Part model, mm, in its own coordinate system. A direction names the side the tool comes from. Give positions to 0.01 mm unless a question says otherwise; leave off trailing zeros. Order: outer loops, then holes, each group sorted by start corner. A loop starts at its lowest first (then second) coordinate and runs counter-clockwise, first axis right, second up. Notation, with made-up numbers: (52.25, 10.5) - (77.25, 10.5) arc R15 cw to (77.25, 28.5) - close; hole circle Ø3 at (49.5, 67.5). An arc over 180 degrees is marked (long way). One line per item, written item: value.
```python
from build123d import *

# Parameters (mm, degrees)
BOSS_EXTRUDE1_DEPTH                  = 194
BOSS_EXTRUDE1_DEPTH_BACK             = 194
TAP_DRILL_FOR_M5X0_8_TAP1_D          = 4.2
TAP_DRILL_FOR_M5X0_8_TAP1_DEPTH      = 3.048
TAP_DRILL_FOR_M3X0_5_TAP1_D          = 2.5
TAP_DRILL_FOR_M3X0_5_TAP1_DEPTH      = 3.048
TAP_DRILL_FOR_M5X0_8_TAP2_AT_2_COUNT = 2
TAP_DRILL_FOR_M5X0_8_TAP2_AT_2_PITCH = 25.4
BOSS_EXTRUDE3_START                  = 40
BOSS_EXTRUDE3_DEPTH                  = 40
M5_CLEARANCE_HOLE1_D                 = 5.3
M5_CLEARANCE_HOLE1_DEPTH             = 3.048
BOSS_EXTRUDE4_START                  = 7
BOSS_EXTRUDE4_DEPTH                  = 7
F_8_0_8_DIAMETER_HOLE1_D             = 8
F_8_0_8_DIAMETER_HOLE1_DEPTH         = 3.048
F_8_0_8_DIAMETER_HOLE2_D             = 8
F_8_0_8_DIAMETER_HOLE2_DEPTH         = 3.048


with BuildPart() as part:
    # Sketch4 → Boss-Extrude1 (new, two sides: drawn at the far end of the back side and taken through both)
    with BuildSketch(Plane(origin=(0, 0, 0), x_dir=(0, 0, -1), z_dir=(1, 0, 0)).offset(-BOSS_EXTRUDE1_DEPTH_BACK)):
        with BuildLine():
            Line((19.05, -17.145), (19.05, 17.145))
            ThreePointArc((19.05, 17.145), (18.492038418, 18.492038418), (17.145, 19.05))
            Line((17.145, 19.05), (-17.145, 19.05))
            ThreePointArc((-17.145, 19.05), (-18.492038418, 18.492038418), (-19.05, 17.145))
            Line((-19.05, 17.145), (-19.05, -17.145))
            ThreePointArc((-19.05, -17.145), (-18.492038418, -18.492038418), (-17.145, -19.05))
            Line((-17.145, -19.05), (17.145, -19.05))
            ThreePointArc((17.145, -19.05), (18.492038418, -18.492038418), (19.05, -17.145))
        make_face()
        with BuildLine():
            Line((16.002, 14.4018), (16.002, -14.4018))
            ThreePointArc((16.002, -14.4018), (15.533312271, -15.533312271), (14.4018, -16.002))
            Line((14.4018, -16.002), (-14.4018, -16.002))
            ThreePointArc((-14.4018, -16.002), (-15.533312271, -15.533312271), (-16.002, -14.4018))
            Line((-16.002, -14.4018), (-16.002, 14.4018))
            ThreePointArc((-16.002, 14.4018), (-15.533312271, 15.533312271), (-14.4018, 16.002))
            Line((-14.4018, 16.002), (14.4018, 16.002))
            ThreePointArc((14.4018, 16.002), (15.533312271, 15.533312271), (16.002, 14.4018))
        make_face(mode=Mode.SUBTRACT)
    extrude(amount=BOSS_EXTRUDE1_DEPTH + BOSS_EXTRUDE1_DEPTH_BACK)

    # Tap Drill for M5x0.8 Tap1
    with Locations(Plane(origin=(0, 19.05, 0), x_dir=(1, 0, 0), z_dir=(0, 1, 0))):
        with Locations((-126, 7.05), (-126, -10.95)):
            tap_drill_for_m5x0_8_tap1 = Hole(TAP_DRILL_FOR_M5X0_8_TAP1_D / 2, depth=TAP_DRILL_FOR_M5X0_8_TAP1_DEPTH)

    # Tap Drill for M3x0.5 Tap1
    with Locations(Plane.XY.offset(19.05)):
        with Locations((149, 9.05), (89, 9.05), (29, 9.05), (-31, 9.05), (-91, 9.05), (-61, 9.05)):
            tap_drill_for_m3x0_5_tap1 = Hole(TAP_DRILL_FOR_M3X0_5_TAP1_D / 2, depth=TAP_DRILL_FOR_M3X0_5_TAP1_DEPTH)

    # Sketch22 → Tap Drill for M5x0.8 Tap2 (revolve, cut)
    with BuildSketch(Plane(origin=(174.95, 12.7, 19.05), x_dir=(0, -1, 0), z_dir=(1, 0, 0))):
        Polygon((0, 0), (0, 6.2618073), (2.1, 5), (2.1, 0), align=None)
    tap_drill_for_m5x0_8_tap2 = revolve(axis=Axis((174.95, 12.7, 25.4), (0, 0, -1)), mode=Mode.SUBTRACT)

    # Tap Drill for M5x0.8 Tap2 at 2: Tap Drill for M5x0.8 Tap2 ×2
    with Locations(*[(0, -i * TAP_DRILL_FOR_M5X0_8_TAP2_AT_2_PITCH, 0) for i in range(1, TAP_DRILL_FOR_M5X0_8_TAP2_AT_2_COUNT)]):
        add(tap_drill_for_m5x0_8_tap2, mode=Mode.SUBTRACT)

    # Mirror1: Tap Drill for M5x0.8 Tap1, Tap Drill for M3x0.5 Tap1, Tap Drill for M5x0.8 Tap2 across plane
    add(tap_drill_for_m5x0_8_tap1.mirror(Plane(origin=(0, 0, 0), x_dir=(0, 0.7071067811865478, 0.7071067811865472), z_dir=(0, -0.7071067811865475, 0.7071067811865477))), mode=Mode.SUBTRACT)
    add(tap_drill_for_m3x0_5_tap1.mirror(Plane(origin=(0, 0, 0), x_dir=(0, 0.7071067811865478, 0.7071067811865472), z_dir=(0, -0.7071067811865475, 0.7071067811865477))), mode=Mode.SUBTRACT)
    add(tap_drill_for_m5x0_8_tap2.mirror(Plane(origin=(0, 0, 0), x_dir=(0, 0.7071067811865478, 0.7071067811865472), z_dir=(0, -0.7071067811865475, 0.7071067811865477))), mode=Mode.SUBTRACT)

    # Mirror1 copy 1 sketch → Mirror1 copy 1 (revolve, cut)
    with BuildSketch(Plane(origin=(174.95, 19.05, -12.7), x_dir=(0, 0, -1), z_dir=(1, 0, 0))):
        Polygon((0, 0), (0, -6.2618073), (2.1, -5), (2.1, 0), align=None)
    revolve(axis=Axis((174.95, 25.4, -12.7), (0, 1, 0)), mode=Mode.SUBTRACT)

    # Sketch11 → Boss-Extrude3 (add)
    with BuildSketch(Plane.ZY.offset(194).offset(BOSS_EXTRUDE3_START)):
        with BuildLine():
            Line((-17.145, -19.05), (17.145, -19.05))
            ThreePointArc((17.145, -19.05), (18.492038418, -18.492038418), (19.05, -17.145))
            Line((19.05, -17.145), (19.05, 17.145))
            ThreePointArc((19.05, 17.145), (18.492038418, 18.492038418), (17.145, 19.05))
            Line((17.145, 19.05), (-17.145, 19.05))
            ThreePointArc((-17.145, 19.05), (-18.492038418, 18.492038418), (-19.05, 17.145))
            Line((-19.05, 17.145), (-19.05, -17.145))
            ThreePointArc((-19.05, -17.145), (-18.492038418, -18.492038418), (-17.145, -19.05))
        make_face()
        with BuildLine():
            Line((-16.002, 14.4018), (-16.002, -14.4018))
            ThreePointArc((-16.002, -14.4018), (-15.533312271, -15.533312271), (-14.4018, -16.002))
            Line((-14.4018, -16.002), (14.4018, -16.002))
            ThreePointArc((14.4018, -16.002), (15.533312271, -15.533312271), (16.002, -14.4018))
            Line((16.002, -14.4018), (16.002, 14.4018))
            ThreePointArc((16.002, 14.4018), (15.533312271, 15.533312271), (14.4018, 16.002))
            Line((14.4018, 16.002), (-14.4018, 16.002))
            ThreePointArc((-14.4018, 16.002), (-15.533312271, 15.533312271), (-16.002, 14.4018))
        make_face(mode=Mode.SUBTRACT)
    extrude(amount=-BOSS_EXTRUDE3_DEPTH)

    # M5 Clearance Hole1
    with Locations(Plane(origin=(0, 19.05, 0), x_dir=(1, 0, 0), z_dir=(0, 1, 0))):
        with Locations((-229, 6.8), (-229, -6.95), (-184, -6.95), (-184, 6.8)):
            m5_clearance_hole1 = Hole(M5_CLEARANCE_HOLE1_D / 2, depth=M5_CLEARANCE_HOLE1_DEPTH)

    # Mirror2: M5 Clearance Hole1 across plane
    add(m5_clearance_hole1.mirror(Plane(origin=(0, 0, 0), x_dir=(0, 0.7071067811865478, 0.7071067811865472), z_dir=(0, -0.7071067811865475, 0.7071067811865477))), mode=Mode.SUBTRACT)

    # Sketch16 → Boss-Extrude4 (add)
    with BuildSketch(Plane.ZY.offset(234).offset(BOSS_EXTRUDE4_START)):
        with BuildLine():
            Line((-17.145, -19.05), (17.145, -19.05))
            ThreePointArc((17.145, -19.05), (18.492038418, -18.492038418), (19.05, -17.145))
            Line((19.05, -17.145), (19.05, 17.145))
            ThreePointArc((19.05, 17.145), (18.492038418, 18.492038418), (17.145, 19.05))
            Line((17.145, 19.05), (-17.145, 19.05))
            ThreePointArc((-17.145, 19.05), (-18.492038418, 18.492038418), (-19.05, 17.145))
            Line((-19.05, 17.145), (-19.05, -17.145))
            ThreePointArc((-19.05, -17.145), (-18.492038418, -18.492038418), (-17.145, -19.05))
        make_face()
        with BuildLine():
            Line((-16.002, 14.4018), (-16.002, -14.4018))
            ThreePointArc((-16.002, -14.4018), (-15.533312271, -15.533312271), (-14.4018, -16.002))
            Line((-14.4018, -16.002), (14.4018, -16.002))
            ThreePointArc((14.4018, -16.002), (15.533312271, -15.533312271), (16.002, -14.4018))
            Line((16.002, -14.4018), (16.002, 14.4018))
            ThreePointArc((16.002, 14.4018), (15.533312271, 15.533312271), (14.4018, 16.002))
            Line((14.4018, 16.002), (-14.4018, 16.002))
            ThreePointArc((-14.4018, 16.002), (-15.533312271, 15.533312271), (-16.002, 14.4018))
        make_face(mode=Mode.SUBTRACT)
    extrude(amount=-BOSS_EXTRUDE4_DEPTH)

    # Ø8.0 (8) Diameter Hole1
    with Locations(Plane.XY.offset(-16.002)):
        with Locations((-229, -6.8), (-229, 6.95), (-184, 6.95), (-184, -6.8)):
            Hole(F_8_0_8_DIAMETER_HOLE1_D / 2, depth=F_8_0_8_DIAMETER_HOLE1_DEPTH)

    # Ø8.0 (8) Diameter Hole2
    with Locations(Plane(origin=(0, -16.002, 0), x_dir=(1, 0, 0), z_dir=(0, 1, 0))):
        with Locations((-229, 6.8), (-229, -6.95), (-184, -6.95), (-184, 6.8)):
            Hole(F_8_0_8_DIAMETER_HOLE2_D / 2, depth=F_8_0_8_DIAMETER_HOLE2_DEPTH)


solid = part.part
```
1) Pin check, flat tips, straight feed: pin 1 (2 mm diameter, centred on x = 149, y = 9.05, fed in from +Z); pin 2 (7 mm diameter, centred on x = -229, y = 6.95, fed in from -Z); pin 3 (7 mm diameter, centred on x = -184, z = 6.95, fed in from -Y). Stop position of each tip, or through.
Outcome:
pin 1: stops at z = -16
pin 2: stops at z = 16
pin 3: stops at y = 16
2) Mould opens along X. For faces 6 (the flat face through (-27, 0, 16.002)), 7 (the flat face through (194, 0, 17)), 8 (the cylindrical face through (-187.815, -17.547, -8.001)) say: released by +X, released by -X, zero draft, split by the parting line, or undercut.
Outcome:
face 6: zero draft
face 7: released by +X
face 8: undercut
3) Drill centre lines: line 1 along Y through (x, z) = (-229, 17); line 2 along Z through (x, y) = (-106.5, 8). Where is each one in solid material? Low to high. Write a range as from..to.
Outcome:
line 1: y = -19.05..-9.45, -4.15..4.3, 9.6..19.05
line 2: z = -19.05..-16, 16..19.05
4) Which spindle directions (+Z, -Z, +X, -X, +Y, -Y) get a long thin tool onto all of the face, cutting with end or side? Do faces 1 (the cylindrical face through (-225, -18, 7)), 2 (the flat face through (-27, -19.05, 0)), 3 (the flat face through (-27, 0, -19.05)), 4 (the cylindrical face through (-225.004, -6.624, -17.547)), 5 (the flat face through (-27, 16.002, 0)). Say none if no direction does.
Outcome:
face 1: -Y
face 2: +Z, -Z, +X, -X, -Y
face 3: -Z, +X, -X, +Y, -Y
face 4: -Z
face 5: +X, -X
5) Cut at A-A, the plane x = 116.5. Give the cut face in (y, z) (3 decimals).
Outcome:
outline: (-19.05, -17.145) arc R1.905 ccw to (-17.145, -19.05) - (17.145, -19.05) arc R1.905 ccw to (19.05, -17.145) - (19.05, 17.145) arc R1.905 ccw to (17.145, 19.05) - (-17.145, 19.05) arc R1.905 ccw to (-19.05, 17.145) - close; hole (-16.002, -14.402) arc R1.6 ccw to (-14.402, -16.002) - (14.402, -16.002) arc R1.6 ccw to (16.002, -14.402) - (16.002, 14.402) arc R1.6 ccw to (14.402, 16.002) - (-14.402, 16.002) arc R1.6 ccw to (-16.002, 14.402) - close
